Geometry check sheet. Reference: the model listing, model coordinates, mm. A direction names the side the tool comes from. Round coordinates to 2 decimals unless told otherwise and drop trailing zeros. Loops run counter-clockwise (first coordinate to the right, second up) from the corner with the lowest first, then second, coordinate; pieces in that order, holes last. Notation, with made-up numbers: M 62.5,7 L 110.5,7 A14 ccw 110.5,13 Z; hole C 17,-21 d2. An arc over 180 degrees is marked long. Use one line per item in the form item = value. Start each with the question number.
1. Cross-section at D-D (x = 3). Record the boundary of the cut face in (y, z).
2. Cross-section at A-A (x = -19.75). Record the boundary of the cut face in (y, z) (3 decimals), then the cut area to 4 significant figures.
3. Material ranges on line 1 (Y direction, x = -19.75, z = 0) (3 decimals); line 2 (Y direction, x = -17, z = 6.25); line 3 (X direction, y = 9, z = 0), recorded low to high.
4. Draft check along X on faces 1 (the flat face through (20.899, 14.532, 4.916)), 2 (the flat face through (-19, 13.75, 4)), 3 (the flat face through (-5.75, -8, 4)), 4 (the cylindrical face through (21.02, -7.37, 0.04)). Enter one of: pulls with the +X half, pulls with the -X half, needs draft (parallel to the pull), parting line crosses it, or undercut.
5. Set-up check for faces 5 (the flat face through (9, 3, 2.5)), 6 (the flat face through (-27.72, 15.27, 4.53)), 7 (the flat face through (-19, -1.5, 4)): record each of +Z, -Z, +X, -X, +Y, -Y from which the full face is reachable in a straight line by a thin tool's end or side.
6. Cross-section at C-C (y = 0). Record the boundary of the cut face in (x, z).
7. Cross-section at B-B (x = 18). Record the boundary of the cut face in (y, z).
8. Go/stop test with flat-tipped pins: pin 1 (4 mm diameter, centred on x = 21, y = 4.5, fed in from +Z); pin 2 (4 mm diameter, centred on x = -19.75, y = 7.625, fed in from +Z); pin 3 (2.5 mm diameter, centred on x = 22, z = -1, fed in from -Y); pin 4 (3 mm diameter, centred on x = 17.5, z = 4.5, fed in from -Y). Record where each tip stops, or that it passes through.
Autodesk Inventor part; units mm, degrees
ref_plane "YZ Plane" through (0, 0, 0) normal (1, 0, 0) x (0, 1, 0)
ref_plane "XZ Plane" through (0, 0, 0) normal (0, 1, 0) x (-1, 0, 0)
ref_plane "XY Plane" through (0, 0, 0) normal (0, 0, 1) x (1, 0, 0)
sketch "Sketch1" plane through (0, 0, 0) normal (0, 0, 1) x (1, 0, 0)
  arc A0 (13.75, 5) -> (13.75, -5) centre (13.75, 0) ccw
  line L0 (29.75, 16.75) -> (-29.75, 16.75)
  line L1 (-29.75, 16.75) -> (-29.75, -16.75)
  line L2 (-29.75, -16.75) -> (29.75, -16.75)
  line L3 (29.75, -16.75) -> (29.75, 16.75)
  line L4 (13.75, 5) -> (29.75, 5)
  line L5 (13.75, -5) -> (29.75, -5)
  arc A1 (13.75, -5) -> (13.75, 5) centre (13.75, 0) ccw construction
  point P0 (0, 0)
  point P1 (0, -16.75)
  point P2 (29.75, 0)
  point P3 (-29.75, 0)
  dimension "d0" = 10
  dimension "d1" = 33.5
  dimension "d2" = 16
  dimension "d3" = 43.5
extrude "Extrusion1" add sketch "Sketch1" along normal mid plane 5 contours A0 L5 L3 L2 L1 L0 L4
sketch "Sketch2" plane through (0, 0, 2.5) normal (0, 0, 1) x (1, 0, 0)
  arc A0 (13.75, 5) -> (13.75, -5) centre (13.75, 0) ccw
  circle A1 centre (5.2647, 8.4853) radius 1.65
  line L0 (13.75, 0) -> (5.2647, 8.4853) construction
  line L1 (13.75, 0) -> (0, 0) construction
  line L2 (13.75, 0) -> (13.75, -13.75) construction
  circle A2 centre (5.2647, -8.4853) radius 1.65
  line L3 (13.75, 0) -> (27.5, 0) construction
  circle A3 centre (22.2353, -8.4853) radius 1.65
  line L4 (13.75, 0) -> (13.75, 13.75) construction
  circle A4 centre (22.2353, 8.4853) radius 1.65
  dimension "d6" = 45
  dimension "d7" = 12
  dimension "d8" = 3.3
  dimension "d11" = 360
extrude "Extrusion2" cut sketch "Sketch2" against normal through all
sketch "Sketch3" plane through (0, 0, 2.5) normal (0, 0, 1) x (1, 0, 0)
  circle A0 centre (-19.75, 7.625) radius 2.1
  line L0 (0, 0) -> (-29.75, 0) construction
  line L1 (-29.75, 16.75) -> (-29.75, -16.75)
  circle A1 centre (-19.75, -7.625) radius 2.1
  dimension "d15" = 4.2
  dimension "d16" = 10
  dimension "d37" = 9.125
extrude "Extrusion3" cut sketch "Sketch3" against normal through all
sketch "Sketch4" plane through (0, 0, 2.5) normal (0, 0, 1) x (1, 0, 0)
  line L0 (-29.75, 16.75) -> (29.75, 16.75)
  line L1 (-29.75, 16.75) -> (29.75, 16.75)
  line L2 (29.75, 16.75) -> (29.75, 13.75)
  line L3 (-29.75, 13.75) -> (-29.75, 16.75)
  line L4 (-2.75, 13.75) -> (-2.75, 0)
  line L5 (-5.75, 1.5) -> (-5.75, 13.75)
  line L6 (-29.75, 1.5) -> (-5.75, 1.5)
  line L7 (-29.75, 0) -> (-29.75, 1.5)
  line L8 (29.75, 13.75) -> (-2.75, 13.75)
  line L9 (-5.75, 13.75) -> (-29.75, 13.75)
  line L10 (0, 0) -> (-29.75, 0) construction
  line L11 (-29.75, -16.75) -> (-29.75, 16.75)
  line L12 (-29.75, -16.75) -> (29.75, -16.75)
  line L13 (-29.75, -16.75) -> (29.75, -16.75)
  line L14 (29.75, -16.75) -> (29.75, -13.75)
  line L15 (-29.75, -13.75) -> (-29.75, -16.75)
  line L16 (-2.75, -13.75) -> (-2.75, 0)
  line L17 (-5.75, -1.5) -> (-5.75, -13.75)
  line L18 (-29.75, -1.5) -> (-5.75, -1.5)
  line L19 (-29.75, 0) -> (-29.75, -1.5)
  line L20 (29.75, -13.75) -> (-2.75, -13.75)
  line L21 (-5.75, -13.75) -> (-29.75, -13.75)
  point P0 (29.75, 5)
  dimension "d20" = 3
  dimension "d21" = 3
  dimension "d23" = 24
  dimension "d24" = 1.5
extrude "Extrusion4" add sketch "Sketch4" along normal blind 4 contours L0 L2 L8 L4 L16 L20 L14 L12 L11 L21 L17 L18 L7 L6 L5 L9 L3
sketch "Sketch5" plane through (0, 0, -2.5) normal (0, 0, -1) x (-1, 0, 0)
  arc A0 (-13.75, -5) -> (-13.75, 5) centre (-13.75, 0) ccw
  line L0 (29.75, 16.75) -> (-29.75, 16.75)
  circle A1 centre (19.75, 7.625) radius 2.1
  circle A2 centre (19.75, -7.625) radius 2.1
  circle A3 centre (-22.2353, -8.4853) radius 1.65
  circle A4 centre (-5.2647, 8.4853) radius 1.65
  circle A5 centre (-5.2647, -8.4853) radius 1.65
  circle A6 centre (-22.2353, 8.4853) radius 1.65
  line L1 (29.75, 16.75) -> (-29.75, 16.75)
  line L2 (-29.75, 16.75) -> (-29.75, 5)
  line L3 (-29.75, 5) -> (-13.75, 5)
  arc A7 (-13.75, -5) -> (-13.75, 5) centre (-13.75, 0) ccw
  line L4 (-13.75, -5) -> (-29.75, -5)
  line L5 (-29.75, -5) -> (-29.75, -16.75)
  line L6 (-29.75, -16.75) -> (29.75, -16.75)
  line L7 (29.75, -16.75) -> (29.75, 16.75)
  line L8 (-13.75, -16.75) -> (-29.75, -16.75)
  line L9 (-29.75, -13.75) -> (-29.75, -5)
  line L10 (-29.75, -5) -> (-29.75, -16.75)
  line L11 (-29.75, 5) -> (-29.75, 16.75)
  line L12 (-13.75, 16.75) -> (-29.75, 16.75)
  arc A8 (-13.75, 16.75) -> (-29.7363, 5) centre (-13.75, 0) ccw
  arc A9 (-29.7363, -5) -> (-13.75, -16.75) centre (-13.75, 0) ccw
  point P0 (0, 0)
extrude "Extrusion5" cut sketch "Sketch5" against normal through all contours A9 L6 L5 L4 | L3 L2 L0 A8
fillet "Fillet1" radius 2 2 edges at (29.7363, -5, 0) (29.7363, 5, 0)
chamfer "Chamfer1" distance 4 angle 45 3 edges at (-29.75, 15.25, 6.5) (-29.75, 0, 6.5) (-29.75, -15.25, 6.5)
sketch "Sketch6" plane through (-29.75, -16.75, -2.5) normal (0, -1, 0) x (1, 0, 0)
  line L0 (58.2436, 5) -> (58.2436, 0)
  line L1 (53.0656, 5) -> (58.2436, 5)
  line L2 (53.0656, 9) -> (53.0656, 5)
  line L3 (43.5, 9) -> (53.0656, 9)
  line L4 (43.5, 9) -> (43.5, 0)
  line L5 (58.2436, 0) -> (43.5, 0)
  line L6 (53.0656, 5) -> (49.0656, 9)
  line L7 (27, 9) -> (53.0656, 9)
  line L8 (53.0656, 9) -> (27, 9)
  line L9 (49.0656, 9) -> (53.0656, 9)
  line L10 (53.0656, 9) -> (53.0656, 5)
  point P0 (29.75, 2.5)
  dimension "d33" = 45
extrude "Extrusion6" cut sketch "Sketch6" against normal through all contours L6 L3 L2
fillet "Fillet2" radius 3 6 edges at (-2.75, -13.75, 4.5) (-5.75, -13.75, 4.5) (-2.75, 13.75, 4.5) (-5.75, -1.5, 4.5) (-5.75, 13.75, 4.5) (-5.75, 1.5, 4.5)
equation "\"d21\" = d20"
equation "\"d24\" = 0.5 * d20"
properties part number "holder-LMF8LUU-z-axis-v2"
Reported:
q1.outline = M -16.75,-2.5 L 16.75,-2.5 L 16.75,6.5 L 13.75,6.5 L 13.75,2.5 L -13.75,2.5 L -13.75,6.5 L -16.75,6.5 Z
q2.outline = M -16.75,-2.5 L -9.725,-2.5 L -9.725,2.5 L -13.75,2.5 L -13.75,6.5 L -16.75,6.5 Z; M -5.525,-2.5 L 5.525,-2.5 L 5.525,2.5 L 1.5,2.5 L 1.5,6.5 L -1.5,6.5 L -1.5,2.5 L -5.525,2.5 Z; M 9.725,-2.5 L 16.75,-2.5 L 16.75,6.5 L 13.75,6.5 L 13.75,2.5 L 9.725,2.5 Z
q2.area = 161.5 mm²
q3.line_1 = -16.75 to -9.725, -5.525 to 5.525, 9.725 to 16.75
q3.line_2 = -16.75 to -13.75, -1.5 to 1.5, 13.75 to 16.75
q3.line_3 = -29.75 to -21.34, -18.16 to 3.7, 6.83 to 20.67, 23.8 to 27.88
q4.face_1 = pulls with the +X half
q4.face_2 = needs draft
q4.face_3 = pulls with the -X half
q4.face_4 = undercut
q5.face_5 = +Z, +X
q5.face_6 = +Z, -X, +Y, -Y
q5.face_7 = +Z, -X
q6.outline = M -29.75,-2.5 L 8.75,-2.5 L 8.75,2.5 L -2.75,2.5 L -2.75,6.5 L -25.75,6.5 L -29.75,2.5 Z
q7.outline = M -16.2,-2.5 L -5,-2.5 L -5,2.5 L -13.75,2.5 L -13.75,6.5 L -16.2,6.5 Z; M 5,-2.5 L 16.2,-2.5 L 16.2,6.5 L 13.75,6.5 L 13.75,2.5 L 5,2.5 Z
q8.pin_1 = 2.5
q8.pin_2 = through
q8.pin_3 = -15.22
q8.pin_4 = -16.6
